Source: CAD feature listing. Evaluate the final solid. Frame: model axes, mm. A direction names the side the tool comes from. Round coordinates to 2 decimals unless told otherwise and drop trailing zeros.
Item 1: Access query for faces 1 (the cylindrical face through (117.82, 8.2, 12.04)), 2 (the flat face through (-5, 13, 15)). Directions: +Z, -Z, +X, -X, +Y, -Y. A direction counts if a zero-diameter tool reaches every point of the face in a straight line with its end or side. Return the directions, or none.
Item 2: First-contact query: P1, Ø1.3, axis at y = 6, z = 10, coming from the -X side; P2, Ø3, axis at x = -2.42, y = 6.55, coming from the -Z side; P3, Ø1.3, axis at y = 5.5, z = 10.5, coming from the +X side; P4, Ø10, axis at x = 112.58, y = 6.55, coming from the +Z side. Flat tips, straight axial feed; report the tip coordinate or a pass-through.
Item 3: Ray query, L1, parallel to X at y = 2.25, z = 7.75; L2, parallel to X at y = 8, z = 9.75; L3, parallel to X at y = 4.25, z = 1.25. Return the intervals inside material, ascending.
Item 4: Pull-direction query (X, two-part tool) for faces 3 (the flat face through (-217.425, 7, 7)), 4 (the flat face through (1, 16.55, 7)), 5 (the cylindrical face through (-112.18, 8.2, 12.04)); classes: released by +X, released by -X, zero draft, split by the parting line, or undercut.
Autodesk Inventor part; units mm, degrees
ref_plane "YZ Plane" through (0, 0, 0) normal (1, 0, 0) x (0, 1, 0)
ref_plane "XZ Plane" through (0, 0, 0) normal (0, 1, 0) x (-1, 0, 0)
ref_plane "XY Plane" through (0, 0, 0) normal (0, 0, 1) x (1, 0, 0)
sketch "Sketch1" plane through (0, 0, 0) normal (0, 0, 1) x (1, 0, 0)
  line L0 (-212.4247, -46.9955) -> (-212.4247, -61.9955)
  line L1 (-212.4247, -61.9955) -> (213.9753, -61.9955)
  line L2 (213.9753, -61.9955) -> (213.9753, -46.9955)
  line L3 (213.9753, -46.9955) -> (-212.4247, -46.9955)
  line L4 (213.9754, 278.5874) -> (243.9754, 278.5874)
  line L5 (243.9754, 278.5874) -> (243.9753, -71.9955)
  line L6 (243.9753, -71.9955) -> (-242.4247, -71.9955)
  line L7 (-242.4247, -71.9955) -> (-242.4246, 278.5875)
  line L8 (-242.4246, 278.5875) -> (-212.4246, 278.5875)
  line L9 (-212.4246, 278.5875) -> (-212.4247, -21.9955)
  line L10 (-212.4247, -21.9955) -> (213.9753, -21.9955)
  line L11 (213.9753, -21.9955) -> (213.9754, 278.5874)
  line L12 (-217.4247, -3.4496) -> (212.5753, -3.4496)
  line L13 (212.5753, -3.4496) -> (212.5753, 16.5504)
  line L14 (212.5753, 16.5504) -> (-217.4247, 16.5504)
  line L15 (-217.4247, 16.5504) -> (-217.4247, -3.4496)
  point P0 (0, 0)
  dimension "d1" = 20
  dimension "d11" = 430
extrude "Extrusion1" add sketch "Sketch1" along normal blind 15 contours L12 L15 L14 L9 | L9 L14 L13 L12
sketch "Sketch2" plane through (0, 0, 0) normal (0, 0, -1) x (-1, 0, 0)
  line L0 (217.4247, -3.4496) -> (-212.5753, -3.4496) construction
  line L1 (2.4247, -3.4496) -> (2.4247, 18.0985) construction
  line L2 (217.4247, 16.5504) -> (217.4247, -3.4496) construction
  line L3 (217.4247, 6.5504) -> (-212.5753, 6.5504) construction
  line L4 (-212.5753, -3.4496) -> (-212.5753, 16.5504) construction
  circle A0 centre (117.4247, 6.5504) radius 2.5
  circle A1 centre (-112.5753, 6.5504) radius 2.5
  circle A2 centre (2.4247, 6.5504) radius 2.5
  point P0 (0, 0)
  dimension "d4" = 5
  dimension "d5" = 100
  dimension "d6" = 5
  dimension "d7" = 100
  dimension "d8" = 5
extrude "Extrusion2" cut sketch "Sketch2" against normal through all
sketch "Sketch3" plane through (0, 0, 15) normal (0, 0, 1) x (1, 0, 0)
  circle A0 centre (-117.4247, 6.5504) radius 2.5
  circle A1 centre (-2.4247, 6.5504) radius 2.5
  circle A2 centre (112.5753, 6.5504) radius 2.5
  circle A3 centre (-117.4247, 6.5504) radius 5.5
  circle A4 centre (-2.4247, 6.5504) radius 5.5
  circle A5 centre (112.5753, 6.5504) radius 5.5
  point P0 (0, 0)
  dimension "d12" = 11
  dimension "d13" = 11
  dimension "d14" = 11
extrude "Extrusion3" cut sketch "Sketch3" against normal blind 6 contours A0 | A1 | A2 | A3 | A4 | A5
sketch "Sketch4" plane through (212.5753, -3.4496, 0) normal (1, 0, 0) x (0, 0, -1)
  circle A0 centre (-11, 10) radius 2.1
  line L0 (-15, 0) -> (-15, 20)
  point P0 (0, 3.4496)
  dimension "d17" = 4.2
  dimension "d18" = 4
extrude "Extrusion4" cut sketch "Sketch4" against normal blind 15
sketch "Sketch5" plane through (-217.4247, -3.4496, 0) normal (-1, 0, 0) x (0, 0, 1)
  circle A0 centre (11, 10) radius 2.1
  circle A1 centre (11, 10) radius 2.1
  point P0 (0, 3.4496)
extrude "Extrusion5" cut sketch "Sketch5" against normal blind 15
sketch "Sketch6" plane through (-217.4247, 16.5504, 0) normal (0, 1, 0) x (1, 0, 0)
  circle A0 centre (65, -7.4061) radius 1.75
  line L0 (430, 0) -> (0, 0) construction
  circle A1 centre (165, -7.4061) radius 1.75
  circle A2 centre (265, -7.4061) radius 1.75
  circle A3 centre (365, -7.4061) radius 1.75
  line L1 (0, 0) -> (0, -15) construction
  point P0 (217.4247, 0)
  dimension "d23" = 3.5
  dimension "d26" = 100
  dimension "d31" = 65
extrude "Extrusion6" cut sketch "Sketch6" against normal through all
properties part number "Wiper Springloaded 1_CPY"
Data:
1. face 1: +Z
1. face 2: +Z, +X, -X, +Y, -Y
2. P1: stops at x = -202.42
2. P2: passes through
2. P3: stops at x = 197.58
2. P4: stops at z = 9
3. L1: x = -217.42 to -154.14, -150.71 to -54.14, -50.71 to 45.86, 49.29 to 145.86, 149.29 to 212.58
3. L2: x = -202.42 to -122.73, -112.12 to -7.73, 2.88 to 107.27, 117.88 to 197.58
3. L3: x = -217.42 to -118.4, -116.45 to -3.4, -1.45 to 111.6, 113.55 to 212.58
4. face 3: released by -X
4. face 4: zero draft
4. face 5: undercut
